Job drawing, mm, ordinate dimensions from the low corner. One solid piece. A direction names the side the tool comes from. Coordinates: 2 decimals unless noted, no trailing zeros. Write each loop counter-clockwise with the first axis right and the second up, starting at its lowest first coordinate (ties: lowest second). Pieces come first, ordered by that corner, then holes.
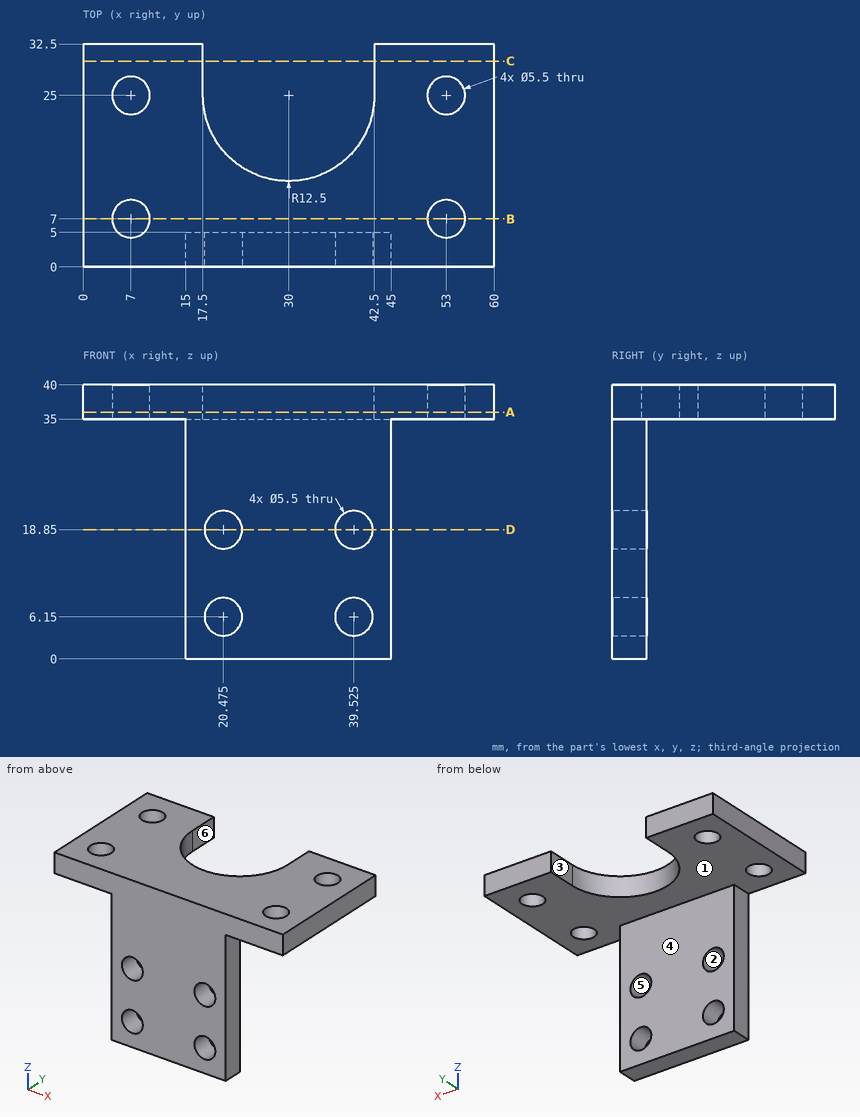
1. Mould opens along Z. For the marked faces 1, 2 and 3 say: +Z half, -Z half, draft (parallel to the pull), parting line (faces both ways), or undercut.
Computed values:
face 1: -Z half
face 2: undercut
face 3: draft
2. Probe line 1 along X through (y, z) = (1.25, 6.15) (3 decimals); line 2 along Y through (x, z) = (53, 37); line 3 along X through (y, z) = (9, 38.5). List the from-to ranges inside material, lowest first.
Computed values:
line 1: x = 15 to 17.725, 23.225 to 36.775, 42.275 to 45
line 2: y = 0 to 4.25, 9.75 to 22.25, 27.75 to 32.5
line 3: x = 0 to 5.11, 8.89 to 51.11, 54.89 to 60
3. Flat gauge pins, fed straight in: pin 1 (4 mm diameter, centred on x = 20, z = 10.5, fed in from +Y); pin 2 (4.5 mm diameter, centred on x = 20.475, z = 18.85, fed in from -Y); pin 3 (12 mm diameter, centred on y = 8, z = 21, fed in from -X); pin 4 (2.5 mm diameter, centred on y = 2, z = 25, fed in from +X). Where does each tip first touch, or does it go through?
Computed values:
pin 1: stops at y = 5
pin 2: passes through
pin 3: stops at x = 15
pin 4: stops at x = 45
4. Saw through at C-C on y = 30. List the corners of the cut face in (x, z), plus the area to 3 significant figures.
Computed values:
outline: (0, 35) - (17.5, 35) - (17.5, 40) - (0, 40) - close; (42.5, 35) - (60, 35) - (60, 40) - (42.5, 40) - close
area: 175 mm2
5. 3-axis set-ups, long thin cutter, end or side, ignore diameter. For the marked faces 4, 5 and 6: which of +Z, -Z, +X, -X, +Y, -Y reach the whole face in a straight line?
Computed values:
face 4: -Z, +X, -X, +Y
face 5: +Y, -Y
face 6: +Z, -Z, +Y
6. Saw through at B-B on y = 7. List the corners of the cut face in (x, z).
Computed values:
outline: (0, 35) - (4.25, 35) - (4.25, 40) - (0, 40) - close; (9.75, 35) - (50.25, 35) - (50.25, 40) - (9.75, 40) - close; (55.75, 35) - (60, 35) - (60, 40) - (55.75, 40) - close
7. Saw through at A-A on z = 36. List the corners of the cut face in (x, y).
Computed values:
outline: (0, 0) - (60, 0) - (60, 32.5) - (42.5, 32.5) - (42.5, 25) arc R12.5 cw to (17.5, 25) - (17.5, 32.5) - (0, 32.5) - close; hole circle Ø5.5 at (7, 7); hole circle Ø5.5 at (7, 25); hole circle Ø5.5 at (53, 7); hole circle Ø5.5 at (53, 25)
8. Saw through at D-D on z = 18.85. List the corners of the cut face in (x, y) (3 decimals), plus the area to 3 significant figures.
Computed values:
outline: (15, 0) - (17.725, 0) - (17.725, 5) - (15, 5) - close; (23.225, 0) - (36.775, 0) - (36.775, 5) - (23.225, 5) - close; (42.275, 0) - (45, 0) - (45, 5) - (42.275, 5) - close
area: 95.0 mm2
